Here's how the part is built. I have some questions about the finished solid (model axes, mm). A direction names the side the tool comes from. Give positions to 0.01 mm unless a question says otherwise; leave off trailing zeros. Loops run counter-clockwise (first coordinate to the right, second up) from the corner with the lowest first, then second, coordinate; pieces in that order, holes last.
Q1. I'm going to push flat-ended pins straight in: P1, Ø2, axis at x = 7, y = -18.5, coming from the -Z side (3 decimals); P2, Ø10, axis at x = -54, y = -48, coming from the -Z side; P3, Ø6, axis at y = -12.5, z = -2, coming from the -X side. Where does each tip first touch, or does it pass through?
Q2. Suppose I cut it at B-B (z = -14). List the corners of the cut face in (x, y) for me.
Q3. I need wall thicknesses on probe 1 along Y at (x, z) = (-24, 26.5); probe 2 along Y at (x, z) = (-13, 53); probe 3 along X at (y, z) = (-29, -10). Which ranges of each line are inside material? Lowest first, please.
Q4. Thinking about a two-plate mould opening in Y: for faces 1 (the face through (-38, -20.857, 53)), 2 (the face through (20.75, -41.9, -12.38)), 3 (the face through (-23, 0, 18)), which applies, pulls with the +Y half, pulls with the -Y half, needs draft (parallel to the pull), parting line crosses it, or undercut?
Q5. For faces 4 (the face through (-53.8, -41.9, -11.7)), 5 (the face through (-24, -42, 15.122)), 6 (the face through (-9, -51, 58.222)), which set-ups out of +Z, -Z, +X, -X, +Y, -Y let a thin tool reach every point of the face, with its end or its side?
Q6. Suppose I cut it at C-C (z = 56). List the corners of the cut face in (x, y) for me, and give its area (3 significant figures).
Q7. Suppose I cut it at D-D (x = 15.5). List the corners of the cut face in (y, z) for me, and give its area (3 significant figures).
```python
from build123d import *

# Parameters (mm, degrees)
F1_DEPTH = 85
F2_R     = 16.36591
F3_DEPTH = 43.1
F4_W     = 22
F4_H     = 12
F5_DEPTH = 11


with BuildPart() as f1:
    # F0 (on Front) → F1 (new body)
    with BuildSketch(Plane.XZ):
        with BuildLine():
            ThreePointArc((-55.954337, 58.221886), (-53.02819, -12.428221), (17.621917, -9.502074))
            Line((17.621917, -9.502074), (23.973947, -15.34886))
            Line((23.973947, -15.34886), (23.973947, 84.758947))
            Line((23.973947, 84.758947), (8.195213, 84.885334))
            Line((8.195213, 84.885334), (7.981639, 58.221886))
            Line((7.981639, 58.221886), (-55.954337, 58.221886))
        make_face()
    extrude(amount=F1_DEPTH)

    # F2 (on face) → F3 (cut)
    with BuildSketch(Plane.XY.offset(58.221886)):
        with Locations((-23.986349, -42.5)):
            Circle(F2_R)
    extrude(amount=-F3_DEPTH, mode=Mode.SUBTRACT)

    # F4 (on face) → F5 (cut)
    with BuildSketch(Plane.XY.offset(58.221886)):
        with Locations((-38.234517, -14.8571)):
            Rectangle(F4_W, F4_H)
    extrude(amount=-F5_DEPTH, mode=Mode.SUBTRACT)


solid = f1.part
```
Solutions:
1. P1: stops at z = -18.845
1. P2: stops at z = -15.76
1. P3: stops at x = -63.37
2. outline: (-51.24, -85) - (12.9, -85) - (12.9, 0) - (-51.24, 0) - close; (22.51, -85) - (23.97, -85) - (23.97, 0) - (22.51, 0) - close
3. probe 1: y = -85 to -58.87, -26.13 to 0
3. probe 2: y = -85 to -54.63, -30.37 to 0
3. probe 3: x = -55.49 to 17.16, 18.16 to 23.97
4. face 1: undercut
4. face 2: needs draft
4. face 3: pulls with the +Y half
5. face 4: +Y, -Y
5. face 5: +Z
5. face 6: +Z, -X, +Y, -Y
6. outline: (-57.88, -85) - (23.97, -85) - (23.97, 0) - (-57.88, 0) - close; hole (-49.23, -20.86) - (-27.23, -20.86) - (-27.23, -8.86) - (-49.23, -8.86) - close; hole circle Ø32.73 at (-23.99, -42.5)
6. area: 5,850 mm2
7. outline: (-85, -11.67) - (0, -11.67) - (0, 84.83) - (-85, 84.83) - close
7. area: 8,200 mm2
